Source: CAD feature listing. Evaluate the final solid. Frame: model axes, mm. Round coordinates to 2 decimals unless told otherwise and drop trailing zeros. Loops run counter-clockwise (first coordinate to the right, second up) from the corner with the lowest first, then second, coordinate; pieces in that order, holes last. Notation, with made-up numbers: (35.25, 7) -> (63.25, 7) arc R20 ccw to (63.25, 45) -> close; hole circle Ø1 at (79, 78). An arc over 180 degrees is marked (long way). Return JSON: item names as keys, results as strings. Group by question number.
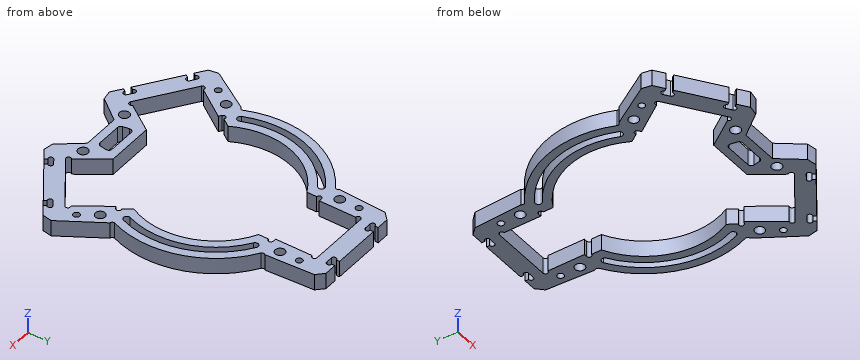
```python
from build123d import *

# Parameters (mm, degrees)
EXTRUDE_1_DEPTH        = 2.5
SKETCH_2_W             = 2.05
SKETCH_2_H             = 5
CUT_EXTRUDE_1_DEPTH    = 6
SKETCH_3_R             = 0.75
CUT_EXTRUDE_2_DEPTH    = 6
CUT_EXTRUDE_3_DEPTH    = 6
SKETCH_5_R             = 0.75
CUT_EXTRUDE_4_DEPTH    = 6
CUT_EXTRUDE_6_DEPTH    = 6
SKETCH_8_R             = 0.75
CUT_EXTRUDE_7_DEPTH    = 6
CUT_EXTRUDE_8_DEPTH    = 6
CUT_EXTRUDE_9_DEPTH    = 6
CUT_EXTRUDE_10_DEPTH   = 6
FILLET_1_R             = 1
SKETCH_12_R            = 1.5
SKETCH_12_R_2          = 1
CUT_EXTRUDE_11_DEPTH   = 6
CHAMFER_1_SIZE2        = 2.113509005
CHAMFER_1_SIZE         = 2
CHAMFER_1_EDGE_2_SIZE2 = 2.113509005
CHAMFER_1_EDGE_2_SIZE  = 2
CHAMFER_1_EDGE_3_SIZE2 = 2
CHAMFER_1_EDGE_3_SIZE  = 2.113509005
CHAMFER_1_EDGE_4_SIZE2 = 2.113509005
CHAMFER_1_EDGE_4_SIZE  = 2
CHAMFER_1_EDGE_5_SIZE2 = 2
CHAMFER_1_EDGE_5_SIZE  = 2.113509005
CHAMFER_1_EDGE_6_SIZE2 = 2.113509005
CHAMFER_1_EDGE_6_SIZE  = 2
SKETCH_13_R            = 1.55
CUT_EXTRUDE_12_DEPTH   = 6


with BuildPart() as part:
    # 草图1 → 凸台-拉伸1 (new body, symmetric)
    with BuildSketch(Plane.XY):
        with BuildLine():
            Line((-15, 49.228571429), (15, 49.228571429))
            Line((15, 49.228571429), (16.242072966, 25.52840738))
            ThreePointArc((16.242072966, 25.52840738), (28.856904848, 9.098547149), (27.947220205, -11.595576762))
            Line((27.947220205, -11.595576762), (40.523629231, -31.722038378))
            Line((40.523629231, -31.722038378), (15.949067902, -48.929331468))
            Line((15.949067902, -48.929331468), (5.796130384, -35.93416405))
            Line((5.796130384, -35.93416405), (-5.796130384, -35.93416405))
            Line((-5.796130384, -35.93416405), (-15.949067902, -48.929331468))
            Line((-15.949067902, -48.929331468), (-40.523629231, -31.722038378))
            Line((-40.523629231, -31.722038378), (-27.947220205, -11.595576762))
            ThreePointArc((-27.947220205, -11.595576762), (-28.856904848, 9.098547149), (-16.242072966, 25.52840738))
            Line((-16.242072966, 25.52840738), (-15, 49.228571429))
        make_face()
        with BuildLine():
            Line((-9.5, 38.228571429), (9.5, 38.228571429))
            Line((9.5, 38.228571429), (9.5, 21.228571429))
            ThreePointArc((9.5, 21.228571429), (22.180886192, 6.993606553), (19.95815277, -11.940451538))
            Line((19.95815277, -11.940451538), (29.708952188, -25.866036291))
            Line((29.708952188, -25.866036291), (14.145063346, -36.763988581))
            Line((14.145063346, -36.763988581), (7.26214611, -26.93416405))
            Line((7.26214611, -26.93416405), (-7.26214611, -26.93416405))
            Line((-7.26214611, -26.93416405), (-14.145063346, -36.763988581))
            Line((-14.145063346, -36.763988581), (-29.708952188, -25.866036291))
            Line((-29.708952188, -25.866036291), (-19.95815277, -11.940451538))
            ThreePointArc((-19.95815277, -11.940451538), (-22.180886192, 6.993606553), (-9.5, 21.228571429))
            Line((-9.5, 21.228571429), (-9.5, 38.228571429))
        make_face(mode=Mode.SUBTRACT)
    extrude(amount=EXTRUDE_1_DEPTH, both=True)

    # 草图2 → 切除-拉伸1 (cut, through all)
    with BuildSketch(Plane.XY.offset(2.5)):
        with Locations((8.425, 43.728571429)):
            Rectangle(SKETCH_2_W, SKETCH_2_H)
        with Locations((-8.425, 43.728571429)):
            Rectangle(SKETCH_2_W, SKETCH_2_H)
        Polygon((34.256606076, -32.447931467), (31.388723894, -28.352171245), (29.709462204, -29.52800294), (32.577344385, -33.623763161), align=None)
        Polygon((15.906750257, -39.192765892), (17.586011948, -38.016934198), (20.45389413, -42.112694419), (18.774632439, -43.288526114), align=None)
        Polygon((-34.256606076, -32.447931467), (-32.577344385, -33.623763161), (-29.709462204, -29.52800294), (-31.388723894, -28.352171245), align=None)
        Polygon((-18.774632439, -43.288526114), (-15.906750257, -39.192765892), (-17.586011948, -38.016934198), (-20.45389413, -42.112694419), align=None)
    extrude(amount=-CUT_EXTRUDE_1_DEPTH, mode=Mode.SUBTRACT)

    # 草图3 → 切除-拉伸2 (cut, through all)
    with BuildSketch(Plane.XY.offset(2.5)):
        with Locations((-9.45, 45.478571429)):
            Circle(SKETCH_3_R)
        with Locations((-9.45, 41.978571429)):
            Circle(SKETCH_3_R)
        with Locations((-7.4, 41.978571429)):
            Circle(SKETCH_3_R)
        with Locations((-7.4, 45.478571429)):
            Circle(SKETCH_3_R)
        with Locations((7.4, 45.478571429)):
            Circle(SKETCH_3_R)
        with Locations((7.4, 41.978571429)):
            Circle(SKETCH_3_R)
        with Locations((9.45, 41.978571429)):
            Circle(SKETCH_3_R)
        with Locations((9.45, 45.478571429)):
            Circle(SKETCH_3_R)
        with Locations((-9.5, 37.478571429)):
            Circle(SKETCH_3_R)
        with Locations((9.5, 37.478571429)):
            Circle(SKETCH_3_R)
        with Locations((-29.27876986, -25.251672257)):
            Circle(SKETCH_3_R)
        with Locations((29.27876986, -25.251672257)):
            Circle(SKETCH_3_R)
        with Locations((-31.818906222, -28.966535279)):
            Circle(SKETCH_3_R)
        with Locations((-30.139644531, -30.142366973)):
            Circle(SKETCH_3_R)
        with Locations((-33.826423749, -31.833567434)):
            Circle(SKETCH_3_R)
        with Locations((-32.147162058, -33.009399128)):
            Circle(SKETCH_3_R)
        with Locations((-18.016194275, -38.631298231)):
            Circle(SKETCH_3_R)
        with Locations((-20.023711803, -41.498330386)):
            Circle(SKETCH_3_R)
        with Locations((-16.336932585, -39.807129926)):
            Circle(SKETCH_3_R)
        with Locations((-18.344450112, -42.674162081)):
            Circle(SKETCH_3_R)
        with Locations((16.336932585, -39.807129926)):
            Circle(SKETCH_3_R)
        with Locations((18.344450112, -42.674162081)):
            Circle(SKETCH_3_R)
        with Locations((18.016194275, -38.631298231)):
            Circle(SKETCH_3_R)
        with Locations((20.023711803, -41.498330386)):
            Circle(SKETCH_3_R)
        with Locations((30.139644531, -30.142366973)):
            Circle(SKETCH_3_R)
        with Locations((32.147162058, -33.009399128)):
            Circle(SKETCH_3_R)
        with Locations((33.826423749, -31.833567434)):
            Circle(SKETCH_3_R)
        with Locations((31.818906222, -28.966535279)):
            Circle(SKETCH_3_R)
        with Locations((-13.714881019, -36.149624548)):
            Circle(SKETCH_3_R)
        with Locations((13.714881019, -36.149624548)):
            Circle(SKETCH_3_R)
    extrude(amount=-CUT_EXTRUDE_2_DEPTH, mode=Mode.SUBTRACT)

    # 草图4 → 切除-拉伸3 (cut, through all)
    with BuildSketch(Plane(origin=(0, 0, -2.5), x_dir=(-1, 0, 0), z_dir=(0, 0, -1))):
        Polygon((-9.5, 25.328571429), (-10.5, 25.328571429), (-10.5, 20.752162415), (-9.5, 21.228571429), align=None)
        Polygon((-22.309816159, -15.298974919), (-23.128968203, -14.725398483), (-20.50404783, -10.976623684), (-19.95815277, -11.940451538), align=None)
        Polygon((20.50404783, -10.976623684), (19.95815277, -11.940451538), (22.309816159, -15.298974919), (23.128968203, -14.725398483), align=None)
        Polygon((10.5, 20.752162415), (9.5, 21.228571429), (9.5, 25.328571429), (10.5, 25.328571429), align=None)
    extrude(amount=-CUT_EXTRUDE_3_DEPTH, mode=Mode.SUBTRACT)

    # 草图5 → 切除-拉伸4 (cut, through all)
    with BuildSketch(Plane(origin=(0, 0, -2.5), x_dir=(-1, 0, 0), z_dir=(0, 0, -1))):
        with Locations((-10.5, 24.578571429)):
            Circle(SKETCH_5_R)
        with Locations((-22.698785876, -14.11103445)):
            Circle(SKETCH_5_R)
        with Locations((22.698785876, -14.11103445)):
            Circle(SKETCH_5_R)
        with Locations((10.5, 24.578571429)):
            Circle(SKETCH_5_R)
    extrude(amount=-CUT_EXTRUDE_4_DEPTH, mode=Mode.SUBTRACT)

    # 草图7 → 切除-拉伸6 (cut, through all)
    with BuildSketch(Plane.XY.offset(2.5)):
        with BuildLine():
            ThreePointArc((-15.041908084, 23.328287396), (-26.472612471, 8.346782651), (-25.702165708, -10.481730275))
            ThreePointArc((-25.702165708, -10.481730275), (-24.398584696, -11.030070084), (-23.850244887, -9.726489073))
            ThreePointArc((-23.850244887, -9.726489073), (-24.565178569, 7.745371052), (-13.958091916, 21.647411876))
            ThreePointArc((-13.958091916, 21.647411876), (-13.65956224, 23.02975772), (-15.041908084, 23.328287396))
        make_face()
        with BuildLine():
            ThreePointArc((15.041908084, 23.328287396), (26.472612471, 8.346782651), (25.702165708, -10.481730275))
            ThreePointArc((25.702165708, -10.481730275), (24.398584696, -11.030070084), (23.850244887, -9.726489073))
            ThreePointArc((23.850244887, -9.726489073), (24.565178569, 7.745371052), (13.958091916, 21.647411876))
            ThreePointArc((13.958091916, 21.647411876), (13.65956224, 23.02975772), (15.041908084, 23.328287396))
        make_face()
    extrude(amount=-CUT_EXTRUDE_6_DEPTH, mode=Mode.SUBTRACT)

    # 草图8 → 切除-拉伸7 (cut, through all)
    with BuildSketch(Plane.XY.offset(2.5)):
        with Locations((-16.644671765, 26.161190287)):
            Circle(SKETCH_8_R)
        with Locations((16.644671765, 26.161190287)):
            Circle(SKETCH_8_R)
        with Locations((-28.639959199, -11.883000989)):
            Circle(SKETCH_8_R)
        with Locations((28.639959199, -11.883000989)):
            Circle(SKETCH_8_R)
    extrude(amount=-CUT_EXTRUDE_7_DEPTH, mode=Mode.SUBTRACT)

    # 草图9 → 切除-拉伸8 (cut, through all)
    with BuildSketch(Plane.XY.offset(2.5)):
        Polygon((-15.288242786, 43.728571429), (15.288242786, 43.728571429), (15, 49.228571429), (-15, 49.228571429), align=None)
    extrude(amount=-CUT_EXTRUDE_8_DEPTH, mode=Mode.SUBTRACT)

    # 草图10 → 切除-拉伸9 (cut, through all)
    with BuildSketch(Plane.XY.offset(2.5)):
        Polygon((-37.605073499, -27.051372864), (-12.558282835, -44.589324495), (-15.949067902, -48.929331468), (-40.523629231, -31.722038378), align=None)
    cut_extrude_9 = extrude(amount=-CUT_EXTRUDE_9_DEPTH, mode=Mode.SUBTRACT)

    # 镜向1: 切除-拉伸9 across plane
    add(cut_extrude_9.mirror(Plane(origin=(0, 0, 0), x_dir=(0, 0, 1), z_dir=(1, 0, 0))), mode=Mode.SUBTRACT)

    # 草图11 → 切除-拉伸10 (cut, through all)
    with BuildSketch(Plane.XY.offset(2.5)):
        Polygon((-5.335149781, -29.43416405), (-4.683587236, -33.43416405), (4.683587236, -33.43416405), (5.335149781, -29.43416405), align=None)
    extrude(amount=-CUT_EXTRUDE_10_DEPTH, mode=Mode.SUBTRACT)

    # 圆角1
    fillet_1_edges = [part.edges().sort_by_distance(p)[0] for p in [
        (-5.335149781, -29.43416405, 0),
        (5.335149781, -29.43416405, 0),
        (4.683587236, -33.43416405, 0),
        (-4.683587236, -33.43416405, 0),
    ]]
    fillet(fillet_1_edges, radius=FILLET_1_R)

    # 草图12 → 切除-拉伸11 (cut, through all)
    with BuildSketch(Plane.XY.offset(2.5)):
        with Locations((-13, 29.228571429)):
            Circle(SKETCH_12_R)
        with Locations((-27.413796415, -16.486150365)):
            Circle(SKETCH_12_R)
        with Locations((13, 29.228571429)):
            Circle(SKETCH_12_R)
        with Locations((27.413796415, -16.486150365)):
            Circle(SKETCH_12_R)
        with Locations((-13, 35.228571429)):
            Circle(SKETCH_12_R_2)
        with Locations((-30.855255033, -21.401062631)):
            Circle(SKETCH_12_R_2)
        with Locations((30.855255033, -21.401062631)):
            Circle(SKETCH_12_R_2)
        with Locations((13, 35.228571429)):
            Circle(SKETCH_12_R_2)
    extrude(amount=-CUT_EXTRUDE_11_DEPTH, mode=Mode.SUBTRACT)

    # 倒角1
    chamfer_1_edges = [part.edges().sort_by_distance(p)[0] for p in [
        (15.288242786, 43.728571429, 0),
    ]]
    chamfer(chamfer_1_edges, length=CHAMFER_1_SIZE, length2=CHAMFER_1_SIZE2)

    # 倒角1 edge 2
    chamfer_1_edge_2_edges = [part.edges().sort_by_distance(p)[0] for p in [
        (-15.288242786, 43.728571429, 0),
    ]]
    chamfer(chamfer_1_edge_2_edges, length=CHAMFER_1_EDGE_2_SIZE, length2=CHAMFER_1_EDGE_2_SIZE2)

    # 倒角1 edge 3
    chamfer_1_edge_3_edges = [part.edges().sort_by_distance(p)[0] for p in [
        (-37.605073499, -27.051372864, 0),
    ]]
    chamfer(chamfer_1_edge_3_edges, length=CHAMFER_1_EDGE_3_SIZE, length2=CHAMFER_1_EDGE_3_SIZE2)

    # 倒角1 edge 4
    chamfer_1_edge_4_edges = [part.edges().sort_by_distance(p)[0] for p in [
        (-12.558282835, -44.589324495, 0),
    ]]
    chamfer(chamfer_1_edge_4_edges, length=CHAMFER_1_EDGE_4_SIZE, length2=CHAMFER_1_EDGE_4_SIZE2)

    # 倒角1 edge 5
    chamfer_1_edge_5_edges = [part.edges().sort_by_distance(p)[0] for p in [
        (12.558282835, -44.589324495, 0),
    ]]
    chamfer(chamfer_1_edge_5_edges, length=CHAMFER_1_EDGE_5_SIZE, length2=CHAMFER_1_EDGE_5_SIZE2)

    # 倒角1 edge 6
    chamfer_1_edge_6_edges = [part.edges().sort_by_distance(p)[0] for p in [
        (37.605073499, -27.051372864, 0),
    ]]
    chamfer(chamfer_1_edge_6_edges, length=CHAMFER_1_EDGE_6_SIZE, length2=CHAMFER_1_EDGE_6_SIZE2)

    # 草图13 → 切除-拉伸12 (cut, through all)
    with BuildSketch(Plane(origin=(0, 0, -2.5), x_dir=(-1, 0, 0), z_dir=(0, 0, -1))):
        with Locations((-9, -35)):
            Circle(SKETCH_13_R)
        with Locations((9, -35)):
            Circle(SKETCH_13_R)
    extrude(amount=-CUT_EXTRUDE_12_DEPTH, mode=Mode.SUBTRACT)


solid = part.part
```
(1) Ray query, line 1 (X direction, y = 32.5, z = -0.9); line 2 (X direction, y = 17, z = -0.9); line 3 (Y direction, x = 8, z = -0.4). Return the intervals inside material, ascending.
(2) Cut plane C-C (y = -8). Return loops of the section in (x, z).
(3) Cut plane B-B (z = -1.3). Count the separate pieces of the cut face and the enclosed holes in it, and give its area (3 significant figures).
(4) Pin query (flat end, axial travel): pin 1 (1.1 mm diameter, centred on y = 43, z = 0.5, fed in from -X); pin 2 (1.1 mm diameter, centred on y = 43.5, z = 0.5, fed in from -X); pin 3 (10 mm diameter, centred on x = 13, y = 12.5, fed in from -Z); pin 4 (3 mm diameter, centred on y = -8, z = -1.5, fed in from +X). Return the tip coordinate at first contact, or that it passes through.
(5) Cut plane A-A (y = 2). Return loops of the section in (x, z), and give its area (3 significant figures).
Answers follow:
{
 "1": {"line 1": "-15.88 to -9.5, 9.5 to 15.88", "line 2": "-25.03 to -21.94, -19.35 to -15.87, 15.87 to 19.35, 21.94 to 25.03", "line 3": "-38.75 to -36.18, -33.82 to -27.99, 38.23 to 41.23"},
 "2": {"outline": "(-29.18, -2.5) -> (-26.58, -2.5) -> (-26.58, 2.5) -> (-29.18, 2.5) -> close; (-24.48, -2.5) -> (-21.84, -2.5) -> (-21.84, 2.5) -> (-24.48, 2.5) -> close; (21.84, -2.5) -> (24.48, -2.5) -> (24.48, 2.5) -> (21.84, 2.5) -> close; (26.58, -2.5) -> (29.18, -2.5) -> (29.18, 2.5) -> (26.58, 2.5) -> close"},
 "3": {"separate pieces": "1", "enclosed holes": "14", "area": "1,360 mm^2"},
 "4": {"pin 1": "x = -14.57", "pin 2": "x = -14.07", "pin 3": "through", "pin 4": "x = 29.55"},
 "5": {"outline": "(-30.19, -2.5) -> (-27.69, -2.5) -> (-27.69, 2.5) -> (-30.19, 2.5) -> close; (-25.68, -2.5) -> (-23.17, -2.5) -> (-23.17, 2.5) -> (-25.68, 2.5) -> close; (23.17, -2.5) -> (25.68, -2.5) -> (25.68, 2.5) -> (23.17, 2.5) -> close; (27.69, -2.5) -> (30.19, -2.5) -> (30.19, 2.5) -> (27.69, 2.5) -> close", "area": "50.1 mm^2"}
}
